Check sheet for the drawn part. Datum: minimum x, y, z corner. Units: mm. A direction names the side the tool comes from. Round coordinates to 2 decimals unless told otherwise and drop trailing zeros. Write each loop counter-clockwise with the first axis right and the second up, starting at its lowest first coordinate (ties: lowest second). Pieces come first, ordered by that corner, then holes. Notation, with made-up numbers: M 68,-5.75 L 75,-5.75 A25 ccw 75,22.25 Z; hole C -12,-11.5 d5. An arc over 180 degrees is marked long. Answer in a Markdown table with one row per item. Add a question column.
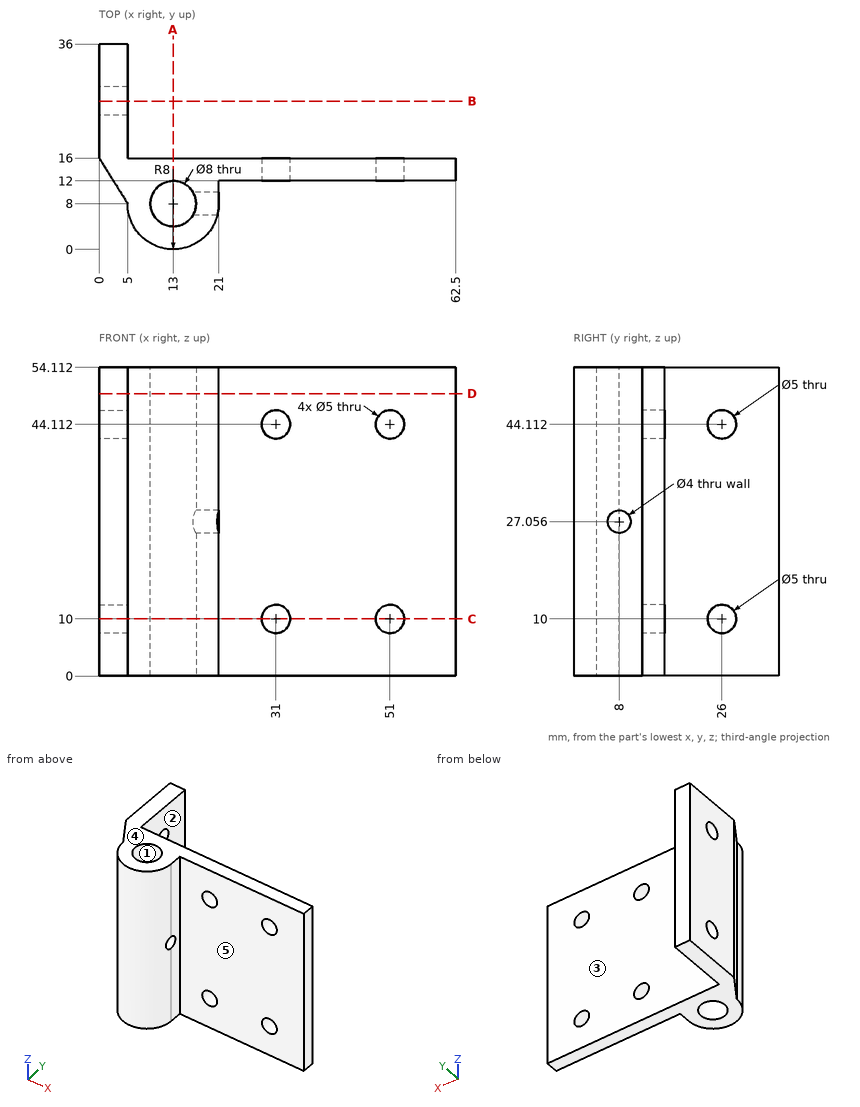
Item 1: Access from +Z, -Z, +X, -X, +Y, -Y to the whole of each face (thin tool, end or side, straight path). Record for the marked faces 4 and 5.
Item 2: Section check D-D, the plane z = 49.5. Record the boundary of the cut face in (x, y).
Item 3: Mould release check, pull along Y, two halves, no side actions. Record for the marked faces 1, 2 and 3: +Y half, -Y half, draft (parallel to the pull), parting line (faces both ways), or undercut.
Item 4: Scan lines: probe 1 along Z at (x, y) = (51, 14.05); probe 2 along Y at (x, z) = (24, 28.5); probe 3 along X at (y, z) = (33, 46). Record each from-to range of solid material in increasing order. Write a range as from..to.
Item 5: Section check C-C, the plane z = 10. Record the boundary of the cut face in (x, y), and give its area (3 significant figures).
Item 6: Gauge pin test, flat ends, axial feed: pin 1 Ø3 at (x, z) = (54.5, 8) entering from -Y; pin 2 Ø6.5 at (y, z) = (8, 27.056) entering from +X; pin 3 Ø10.5 at (x, y) = (13, 8) entering from +Z; pin 4 Ø8 at (y, z) = (26, 44.112) entering from +X. Record the tip position at first contact, or that the pin passes through.
Item 7: Section check A-A, the plane x = 13. Record the boundary of the cut face in (y, z), and give its area (3 significant figures).
Item 8: Section check B-B, the plane y = 26. Record the boundary of the cut face in (x, z), and give its area (3 significant figures).
Result sheet:
| question | item | result |
|---|---|---|
| 1 | face 4 | +Z, +X, -X, +Y, -Y |
| 1 | face 5 | +Z, -Z, +X, -Y |
| 2 | outline | M 0,16 L 5,8 A8 ccw 21,8 L 21,12 L 62.5,12 L 62.5,16 L 5,16 L 5,36 L 0,36 Z; hole C 13,8 d8 |
| 3 | face 1 | undercut |
| 3 | face 2 | draft |
| 3 | face 3 | +Y half |
| 4 | probe 1 | z = 0..7.5, 12.5..41.61, 46.61..54.11 |
| 4 | probe 2 | y = 12..16 |
| 4 | probe 3 | x = 0..5 |
| 5 | outline | M 0,16 L 5,8 A8 ccw 21,8 L 21,12 L 28.5,12 L 28.5,16 L 5,16 L 5,23.5 L 0,23.5 Z; M 0,28.5 L 5,28.5 L 5,36 L 0,36 Z; M 33.5,12 L 48.5,12 L 48.5,16 L 33.5,16 Z; M 53.5,12 L 62.5,12 L 62.5,16 L 53.5,16 Z; hole C 13,8 d8 |
| 5 | area | 399 mm^2 |
| 6 | pin 1 | stops at y = 12 |
| 6 | pin 2 | stops at x = 21 |
| 6 | pin 3 | stops at z = 54.11 |
| 6 | pin 4 | stops at x = 5 |
| 7 | outline | M 0,0 L 4,0 L 4,54.11 L 0,54.11 Z; M 12,0 L 16,0 L 16,54.11 L 12,54.11 Z |
| 7 | area | 433 mm^2 |
| 8 | outline | M 0,0 L 5,0 L 5,7.5 L 0,7.5 Z; M 0,12.5 L 5,12.5 L 5,41.61 L 0,41.61 Z; M 0,46.61 L 5,46.61 L 5,54.11 L 0,54.11 Z |
| 8 | area | 221 mm^2 |
